```python
from build123d import *

# Parameters (mm, degrees)
SKETCH_1_R      = 1.35
SKETCH_1_R_2    = 5.1
EXTRUDE_1_DEPTH = 3


with BuildPart() as part:
    # 草图1 → 凸台-拉伸1 (new body)
    with BuildSketch(Plane.XY):
        with BuildLine():
            Line((-14, 0), (-14, 150))
            ThreePointArc((-14, 150), (0, 164), (14, 150))
            Line((14, 150), (14, 0))
            ThreePointArc((14, 0), (0, -14), (-14, 0))
        make_face()
        with Locations((0, 161)):
            Circle(SKETCH_1_R, mode=Mode.SUBTRACT)
        with Locations((7.778174593, 157.778174593)):
            Circle(SKETCH_1_R, mode=Mode.SUBTRACT)
        with Locations((11, 150)):
            Circle(SKETCH_1_R, mode=Mode.SUBTRACT)
        with Locations((7.778174593, 142.221825407)):
            Circle(SKETCH_1_R, mode=Mode.SUBTRACT)
        with Locations((0, 139)):
            Circle(SKETCH_1_R, mode=Mode.SUBTRACT)
        with Locations((-7.778174593, 142.221825407)):
            Circle(SKETCH_1_R, mode=Mode.SUBTRACT)
        with Locations((-11, 150)):
            Circle(SKETCH_1_R, mode=Mode.SUBTRACT)
        with Locations((-7.778174593, 157.778174593)):
            Circle(SKETCH_1_R, mode=Mode.SUBTRACT)
        with Locations((0, 150)):
            Circle(SKETCH_1_R_2, mode=Mode.SUBTRACT)
        Circle(SKETCH_1_R_2, mode=Mode.SUBTRACT)
        with Locations((0, -11)):
            Circle(SKETCH_1_R, mode=Mode.SUBTRACT)
        with Locations((-7.778174593, -7.778174593)):
            Circle(SKETCH_1_R, mode=Mode.SUBTRACT)
        with Locations((-11, 0)):
            Circle(SKETCH_1_R, mode=Mode.SUBTRACT)
        with Locations((-7.778174593, 7.778174593)):
            Circle(SKETCH_1_R, mode=Mode.SUBTRACT)
        with Locations((0, 11)):
            Circle(SKETCH_1_R, mode=Mode.SUBTRACT)
        with Locations((7.778174593, 7.778174593)):
            Circle(SKETCH_1_R, mode=Mode.SUBTRACT)
        with Locations((11, 0)):
            Circle(SKETCH_1_R, mode=Mode.SUBTRACT)
        with Locations((7.778174593, -7.778174593)):
            Circle(SKETCH_1_R, mode=Mode.SUBTRACT)
    extrude(amount=EXTRUDE_1_DEPTH)


solid = part.part
```
Geometry check sheet. Reference: the model listing, model coordinates, mm. Give positions to 0.01 mm unless a question says otherwise; leave off trailing zeros.
1. Thickness scan on L1, parallel to Y at x = 7.25, z = 1.65; L2, parallel to Y at x = -6.75, z = 0.5; L3, parallel to Y at x = 11, z = 2.35. Record the ranges inside material, lowest first.
2. Section check A-A, the plane z = 2.05. Give the number of separate pieces and of enclosed holes in the cut face, and give its area (3 significant figures).
3. Gauge pin test, flat end, axial feed: pin 1 Ø2.5 at (x, y) = (7.78, 142.22) entering from -Z. Record the tip position at first contact, or that the pin passes through.
4. Release check for a two-part mould opening along Y. For faces 1 (the face through (-14, 74, 1)), 2 (the face through (2.4, -4.5, 1.5)), 3 (the face through (0, 164, 1)) record: pulls with the +Y half, pulls with the -Y half, needs draft (parallel to the pull), parting line crosses it, or undercut.
Values follow:
1. L1: y = -11.98 to -9.02, -6.54 to 6.54, 9.02 to 140.98, 143.46 to 156.54, 159.02 to 161.98
1. L2: y = -12.27 to -8.65, -6.9 to 6.9, 8.65 to 141.35, 143.1 to 156.9, 158.65 to 162.27
1. L3: y = -8.66 to -1.35, 1.35 to 148.65, 151.35 to 158.66
2. separate pieces: 1
2. enclosed holes: 18
2. area: 4,560 mm2
3. pin 1: passes through
4. face 1: needs draft
4. face 2: undercut
4. face 3: pulls with the +Y half
